from build123d import *

# Parameters (mm, degrees)
F0_W     = 16.51
F0_H     = 19.05
F0_W_2   = 13.9302
F0_H_2   = 1.930798
F0_H_3   = 1.311754
F0_H_4   = 1.36334
F0_H_5   = 1.430876
F0_H_6   = 1.339917
F0_H_7   = 1.881583
F1_DEPTH = 3.175
F2_R     = 0.254


with BuildPart() as f1:
    # F0 (on Top) → F1 (new body)
    with BuildSketch(Plane.XY):
        with Locations((0.161979, -0.164203)):
            Rectangle(F0_W, F0_H)
        with Locations((0.161979, -8.088804)):
            Rectangle(F0_W_2, F0_H_2, mode=Mode.SUBTRACT)
        with Locations((0.161979, -5.249125)):
            Rectangle(F0_W_2, F0_H_3, mode=Mode.SUBTRACT)
        with Locations((0.161979, -2.673489)):
            Rectangle(F0_W_2, F0_H_4, mode=Mode.SUBTRACT)
        Polygon((-6.803121, 0.538338), (7.127079, 0.538338), (7.127079, -0.876588), (-6.803121, -0.876588), (-6.803121, -0.164203), align=None, mode=Mode.SUBTRACT)
        with Locations((0.161979, 2.388693)):
            Rectangle(F0_W_2, F0_H_5, mode=Mode.SUBTRACT)
        with Locations((0.161979, 4.85742)):
            Rectangle(F0_W_2, F0_H_6, mode=Mode.SUBTRACT)
        with Locations((0.161979, 7.785006)):
            Rectangle(F0_W_2, F0_H_7, mode=Mode.SUBTRACT)
    extrude(amount=F1_DEPTH)

    # F2
    f2_edges = [f1.edges().sort_by_distance(p)[0] for p in [
        (-8.093021, -0.164203, 3.175),
        (0.161979, -9.689203, 3.175),
        (8.416979, -0.164203, 3.175),
        (0.161979, 9.360797, 3.175),
        (-6.803121, -8.088804, 3.175),
        (0.161979, -7.123405, 3.175),
        (7.127079, -8.088804, 3.175),
        (0.161979, -9.054203, 3.175),
        (0.161979, -4.593248, 3.175),
        (7.127079, -5.249125, 3.175),
        (0.161979, -5.905002, 3.175),
        (-6.803121, -5.249125, 3.175),
        (0.161979, -1.991819, 3.175),
        (7.127079, -2.673489, 3.175),
        (0.161979, -3.355159, 3.175),
        (-6.803121, -2.673489, 3.175),
        (0.161979, 0.538338, 3.175),
        (7.127079, -0.169125, 3.175),
        (0.161979, -0.876588, 3.175),
        (-6.803121, -0.169125, 3.175),
        (-6.803121, 2.388693, 3.175),
        (0.161979, 3.104131, 3.175),
        (7.127079, 2.388693, 3.175),
        (0.161979, 1.673255, 3.175),
        (0.161979, 5.527379, 3.175),
        (7.127079, 4.857421, 3.175),
        (0.161979, 4.187462, 3.175),
        (-6.803121, 4.857421, 3.175),
        (7.127079, 7.785005, 3.175),
        (0.161979, 6.844214, 3.175),
        (-6.803121, 7.785005, 3.175),
        (0.161979, 8.725797, 3.175),
    ]]
    fillet(f2_edges, radius=F2_R)


solid = f1.part
Could you check a few things on this model? Use its own coordinates, in mm. A direction names the side the tool comes from. Give positions to 0.01 mm unless a question says otherwise; leave off trailing zeros. Write each loop counter-clockwise with the first axis right and the second up, starting at its lowest first coordinate (ties: lowest second). Pieces come first, ordered by that corner, then holes. Notation, with made-up numbers: (-25.5, 19) - (5.5, 19) arc R26 cw to (5.5, 51) - close; hole circle Ø5 at (30, -26). An arc over 180 degrees is marked (long way). Use CSV: the item, a comma, the result in double quotes. Start each with the question number.
Item 1: I want a section at A-A, the plane y = -2.25. Please give me the cut outline in (x, z) (3 decimals), then the cut area to 3 significant figures.
Item 2: If we mould it in two halves opening along X, with no side actions, what happens to faces 3 (the face through (8.417, 0, 1)), 4 (the face through (-2, -4, 3.175)), 5 (the face through (0, -5.905, 1))? For each: pulls with the +X half, pulls with the -X half, needs draft (parallel to the pull), parting line crosses it, or undercut.
Item 3: For faces 1 (the face through (0, -4, 0)), 2 (the face through (0, 8.726, 1)), which set-ups out of +Z, -Z, +X, -X, +Y, -Y let a thin tool reach every point of the face, with its end or its side?
Item 4: I want a section at B-B, the plane z = 0.9. Give the number of separate pieces and of enclosed holes in the cut face, then the cut area to 3 significant figures.
Item 5: If I drill on line 1 along X through (y, z) = (8, 2.1); line 2 along Z through (x, y) = (4.25, 4), over which ranges is the centre line in solid material (lowest first)?
Findings:
1,outline,"(-8.093, 0) - (-6.803, 0) - (-6.803, 2.921) arc R0.254 ccw to (-7.057, 3.175) - (-7.839, 3.175) arc R0.254 ccw to (-8.093, 2.921) - close; (7.127, 0) - (8.417, 0) - (8.417, 2.921) arc R0.254 ccw to (8.163, 3.175) - (7.381, 3.175) arc R0.254 ccw to (7.127, 2.921) - close"
1,area,"8.14 mm2"
2,face 3,"pulls with the +X half"
2,face 4,"needs draft"
2,face 5,"undercut"
3,face 1,"-Z, +X, -X, +Y, -Y"
3,face 2,"+Z, -Z"
4,separate pieces,"1"
4,enclosed holes,"7"
4,area,"166 mm2"
5,line 1,"x = -8.09 to -6.8, 7.13 to 8.42"
5,line 2,"z = 0 to 3.17"
